from build123d import *

# Parameters (mm, degrees)
SKETCH1_R           = 2.499798637
BOSS_EXTRUDE1_DEPTH = 3.175
FILLET1_R           = 1


with BuildPart() as part:
    # Sketch1 → Boss-Extrude1 (new body)
    with BuildSketch(Plane(origin=(0, 0, 0), x_dir=(1, 0, 0), z_dir=(0, 1, 0))):
        with BuildLine():
            Line((-67.701379439, -26.588630041), (-118.732469461, -26.59066957))
            ThreePointArc((-118.732469461, -26.59066957), (-122.268132547, -25.126274131), (-123.732669293, -21.590669574))
            Line((-123.732669293, -21.590669574), (-123.732669293, 19.553345865))
            ThreePointArc((-123.732669293, 19.553345865), (-122.268209036, 23.088873934), (-118.732685802, 24.553345865))
            Line((-118.732685802, 24.553345865), (-67.702190036, 24.553514364))
            ThreePointArc((-67.702190036, 24.553514364), (-64.166670991, 23.08907964), (-62.702173527, 19.553586583))
            Line((-62.702173527, 19.553586583), (-62.701579271, -21.588557825))
            ThreePointArc((-62.701579271, -21.588557825), (-64.165949181, -25.124067765), (-67.701379439, -26.588630041))
        make_face()
        with Locations((-118.217169293, 18.981347567)):
            Circle(SKETCH1_R, mode=Mode.SUBTRACT)
        with Locations((-68.217665265, 18.981512662)):
            Circle(SKETCH1_R, mode=Mode.SUBTRACT)
        with Locations((-68.217087532, -21.016650648)):
            Circle(SKETCH1_R, mode=Mode.SUBTRACT)
        with Locations((-118.217169293, -21.018648971)):
            Circle(SKETCH1_R, mode=Mode.SUBTRACT)
    extrude(amount=BOSS_EXTRUDE1_DEPTH)

    # Fillet1
    fillet1_edges = [part.edges().sort_by_distance(p)[0] for p in [
        (-122.268132547, 3.175, 25.126274131),
        (-123.732669293, 0, 1.018661855),
        (-122.268209036, 0, -23.088873934),
        (-93.21692445, 3.175, 26.589649806),
        (-64.165949181, 3.175, 25.124067765),
        (-62.701876399, 3.175, 1.017485621),
        (-64.166670991, 3.175, -23.08907964),
        (-93.217437919, 3.175, -24.553430114),
        (-122.268209036, 3.175, -23.088873934),
        (-123.732669293, 3.175, 1.018661855),
        (-93.217437919, 0, -24.553430114),
        (-64.166670991, 0, -23.08907964),
        (-62.701876399, 0, 1.017485621),
        (-64.165949181, 0, 25.124067765),
        (-93.21692445, 0, 26.589649806),
        (-122.268132547, 0, 25.126274131),
    ]]
    fillet(fillet1_edges, radius=FILLET1_R)


solid = part.part
Build history of the part. All positions in model axes, mm. Round coordinates to 2 decimals unless told otherwise and drop trailing zeros. Write each loop counter-clockwise with the first axis right and the second up, starting at its lowest first coordinate (ties: lowest second). Pieces come first, ordered by that corner, then holes. Notation, with made-up numbers: (44.5, 80) - (67.5, 80) arc R24 cw to (67.5, 109) - close; hole circle Ø2 at (75, 16.25). An arc over 180 degrees is marked (long way). One line per question, with ' | ' between items.
1. Drill centre lines: line 1 along Z through (x, y) = (-118, 0.9); line 2 along Z through (x, y) = (-68, 0.5); line 3 along Z through (x, y) = (-79.5, 1.2). Where is each one in solid material? Low to high. Write a range as from..to.
Results are:
line 1: -24.55..-21.47, -16.49..18.53, 23.51..26.59 | line 2: -24.42..-21.47, -16.49..18.53, 23.51..26.45 | line 3: -24.55..26.59
2. Drop a flat-ended pin along its axis: pin 1 Ø4 at (x, z) = (-68.22, -18.98) entering from +Y. Give the stop position or say it passes through.
Results are:
pin 1: through
3. Band-saw the part on B-B, the plane z = -18. Give the number of separate pieces and of enclosed holes in the cut face, and give its area (3 significant figures).
Results are:
separate pieces: 3 | enclosed holes: 0 | area: 164 mm^2
4. Band-saw the part on A-A, the plane y = 1.5. Write the cut outline in (x, z).
Results are:
outline: (-123.73, -19.55) arc R5 ccw to (-118.73, -24.55) - (-67.7, -24.55) arc R5 ccw to (-62.7, -19.55) - (-62.7, 21.59) arc R5 ccw to (-67.7, 26.59) - (-118.73, 26.59) arc R5 ccw to (-123.73, 21.59) - close; hole circle Ø5 at (-118.22, -18.98); hole circle Ø5 at (-118.22, 21.02); hole circle Ø5 at (-68.22, -18.98); hole circle Ø5 at (-68.22, 21.02)
5. Mould opens along X. For faces 1 (the face through (-64.21, 1.58, -23.13)), 2 (the face through (-117.064, 1.565, -16.764)), 3 (the face through (-68.543, 1.565, 18.538)), 4 (the face through (-122.307, 1.579, -23.05)) say: released by +X, released by -X, zero draft, split by the parting line, or undercut.
Results are:
face 1: released by +X | face 2: undercut | face 3: undercut | face 4: released by -X
